Input: part model. Units: mm. Frame: model coordinates. Face numbers are marked on the shaded views. A direction names the side the tool comes from. Coordinates: 2 decimals unless noted, no trailing zeros. Loops run counter-clockwise (first coordinate to the right, second up) from the corner with the lowest first, then second, coordinate; pieces in that order, holes last. Notation, with made-up numbers: (6.25, 8.5) -> (26.25, 8.5) arc R32 ccw to (26.25, 34.5) -> close; hole circle Ø10 at (-33.5, 16). An arc over 180 degrees is marked (long way). Put each result on its own line as item: value. Start each with the question number.
1) Cut plane A-A (z = 41.5). Return the cut outline in (x, y).
2) Set-up query: the marked faces 5, 6, 7 and 8. Return all of +Z, -Z, +X, -X, +Y, -Y with unobstructed straight access to the full face (end or side cutting, diameter ignored); none if empty.
3) Cut plane B-B (y = -7.25). Return the cut outline in (x, z), plus the area to 3 significant figures.
4) Cut plane D-D (z = 15). Return the cut outline in (x, y), plus the area to 3 significant figures.
5) Pull-direction query (X, two-part tool) for the marked faces 1, 2, 3 and 4; classes: pulls with the +X half, pulls with the -X half, needs draft (parallel to the pull), parting line crosses it, or undercut.
6) Contact query for flat-ended pins moving along their axis: P1, Ø3.5, axis at x = 37.5, z = 49, coming from the -Y side; P2, Ø3, axis at x = -28.5, y = -5, coming from the +Z side; P3, Ø10, axis at x = 39, y = 6.5, coming from the +Z side; P4, Ø3, axis at x = 42, z = 75, coming from the +Y side. Output: stop coordinate, or through.
7) Material intervals for L1, parallel to X at y = -3, z = 32; L2, parallel to X at y = 0.5, z = 72; L3, parallel to Y at x = 36.5, z = 35, sorted ascending.
8) Cut plane C-C (y = 11.25). Return the cut outline in (x, z).
from build123d import *

# Parameters (mm, degrees)
BOSS_EXTRU_1_DEPTH      = 68
ENL_V_MAT_EXTRU_1_DEPTH = 30
BOSS_EXTRU_2_DEPTH      = 10


with BuildPart() as part:
    # Esquisse1 → Boss.-Extru.1 (new body)
    with BuildSketch(Plane.XY):
        Polygon((-32.503867199, -5.5), (-32.503867199, -10.5), (-35.503867199, -10.5), (-35.503867199, 12.2), (45.496132801, 12.2), (45.496132801, -10.5), (42.496132801, -10.5), (42.496132801, -5.5), (35.496132801, -5.5), (35.496132801, 0), (-25.503867199, 0), (-25.503867199, -5.5), align=None)
    extrude(amount=BOSS_EXTRU_1_DEPTH)

    # Esquisse2 → Enlèv. mat.-Extru.1 (cut)
    with BuildSketch(Plane(origin=(0, 12.2, 0), x_dir=(1, 0, 0), z_dir=(0, 1, 0))):
        with BuildLine():
            Line((-25.003867199, -34), (-25.003867199, -68))
            Line((-25.003867199, -68), (34.996132801, -68))
            Line((34.996132801, -68), (34.996132801, -34))
            ThreePointArc((34.996132801, -34), (4.996132801, -4), (-25.003867199, -34))
        make_face()
    extrude(amount=-ENL_V_MAT_EXTRU_1_DEPTH, mode=Mode.SUBTRACT)

    # Esquisse3 → Boss.-Extru.2 (add)
    with BuildSketch(Plane.XY.offset(68)):
        Polygon((-35.503867199, -3.7), (-35.503867199, 3), (-25.003867199, 3), (-25.003867199, 0), (-25.503867199, 0), (-25.503867199, -0.338080905), align=None)
        Polygon((35.496132801, -0.338080905), (35.496132801, 0), (34.996132801, 0), (34.996132801, 3), (45.496132801, 3), (45.496132801, -3.7), align=None)
    extrude(amount=BOSS_EXTRU_2_DEPTH)


solid = part.part
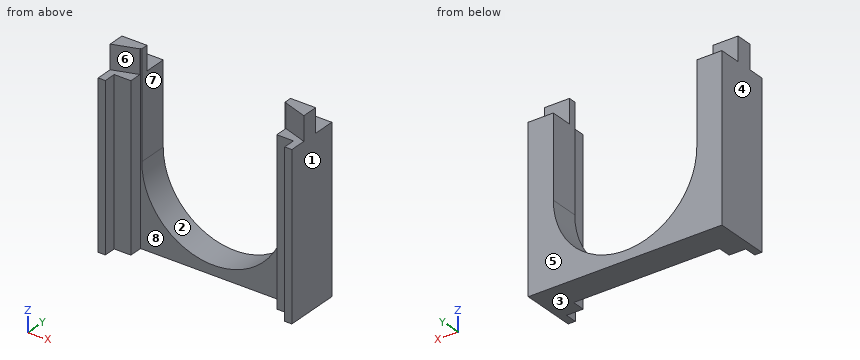
Results found:
1. outline: (-35.5, -10.5) -> (-32.5, -10.5) -> (-32.5, -5.5) -> (-25.5, -5.5) -> (-25.5, 0) -> (-25, 0) -> (-25, 12.2) -> (-35.5, 12.2) -> close; (35, 0) -> (35.5, 0) -> (35.5, -5.5) -> (42.5, -5.5) -> (42.5, -10.5) -> (45.5, -10.5) -> (45.5, 12.2) -> (35, 12.2) -> close
2. face 5: +Z, -Z, +X, -X, +Y
2. face 6: +Z, -Y
2. face 7: +Z, +Y, -Y
2. face 8: +Z, -Z, -Y
3. outline: (-35.5, 0) -> (-32.5, 0) -> (-32.5, 68) -> (-35.5, 68) -> close; (42.5, 0) -> (45.5, 0) -> (45.5, 68) -> (42.5, 68) -> close
3. area: 408 mm2
4. outline: (-35.5, -10.5) -> (-32.5, -10.5) -> (-32.5, -5.5) -> (-25.5, -5.5) -> (-25.5, 0) -> (-18.22, 0) -> (-18.22, 12.2) -> (-35.5, 12.2) -> close; (28.21, 0) -> (35.5, 0) -> (35.5, -5.5) -> (42.5, -5.5) -> (42.5, -10.5) -> (45.5, -10.5) -> (45.5, 12.2) -> (28.21, 12.2) -> close
4. area: 562 mm2
5. face 1: pulls with the +X half
5. face 2: undercut
5. face 3: needs draft
5. face 4: pulls with the -X half
6. P1: stops at y = -5.5
6. P2: stops at z = 68
6. P3: stops at z = 78
6. P4: stops at y = 3
7. L1: x = -35.5 to -25.5, 35.5 to 45.5
7. L2: x = -35.5 to -25, 35 to 45.5
7. L3: y = -5.5 to 12.2
8. outline: (-35.5, 0) -> (45.5, 0) -> (45.5, 68) -> (35, 68) -> (35, 34) arc R30 cw to (-25, 34) -> (-25, 68) -> (-35.5, 68) -> close
